from build123d import *

# Parameters (mm, degrees)
SKETCH1_W           = 260.096
SKETCH1_H           = 179.705
SKETCH1_W_2         = 1.524
SKETCH1_H_2         = 1.016
SKETCH1_W_3         = 1.3716
SKETCH1_W_4         = 1.397
SKETCH1_R           = 1.143
BOSS_EXTRUDE1_DEPTH = 3.048
BOSS_EXTRUDE2_DEPTH = 32.5374
SKETCH1_6_R         = 2.7686
SKETCH1_6_R_2       = 1.8415
BOSS_EXTRUDE3_DEPTH = 7.0104
BOSS_EXTRUDE4_DEPTH = 4.064
SKETCH1_8_R         = 3.9624
SKETCH1_8_R_2       = 1.651
BOSS_EXTRUDE5_DEPTH = 21.844
SKETCH3_W           = 254
SKETCH3_H           = 1.778
CUT_EXTRUDE1_DEPTH  = 0.508


# Read off the part's stored shape, not the designer's step: Boss-Extrude2
with BuildPart() as part:
    # Sketch1 → Boss-Extrude1 (new body)
    with BuildSketch(Plane.XY):
        Rectangle(SKETCH1_W, SKETCH1_H)
        with Locations((-126.238, -85.6615)):
            Rectangle(SKETCH1_W_2, SKETCH1_H_2, mode=Mode.SUBTRACT)
        with Locations((-126.3142, -58.2676)):
            Rectangle(SKETCH1_W_3, SKETCH1_H_2, mode=Mode.SUBTRACT)
        with Locations((-126.3142, -55.2704)):
            Rectangle(SKETCH1_W_3, SKETCH1_H_2, mode=Mode.SUBTRACT)
        with Locations((-126.3015, -20.4216)):
            Rectangle(SKETCH1_W_4, SKETCH1_H_2, mode=Mode.SUBTRACT)
        with Locations((-126.3015, -17.4244)):
            Rectangle(SKETCH1_W_4, SKETCH1_H_2, mode=Mode.SUBTRACT)
        with Locations(Location((-113.9952, -68.9864, 0), (0, 0, 180))):
            Circle(SKETCH1_R, mode=Mode.SUBTRACT)
        with Locations((-126.3015, 17.4244)):
            Rectangle(SKETCH1_W_4, SKETCH1_H_2, mode=Mode.SUBTRACT)
        with Locations((-126.3015, 20.4216)):
            Rectangle(SKETCH1_W_4, SKETCH1_H_2, mode=Mode.SUBTRACT)
        with Locations((-126.3015, 55.2704)):
            Rectangle(SKETCH1_W_4, SKETCH1_H_2, mode=Mode.SUBTRACT)
        with Locations((-126.3015, 58.2676)):
            Rectangle(SKETCH1_W_4, SKETCH1_H_2, mode=Mode.SUBTRACT)
    extrude(amount=BOSS_EXTRUDE1_DEPTH)

    # Boss-Extrude2 outline → Boss-Extrude2 (add)
    with BuildSketch(Plane.XY):
        Polygon((-127, -87.9475), (-127, -86.1695), (-125.476, -86.1695), (-125.476, -85.1535), (-127, -85.1535), (-127, 85.1535), (-125.476, 85.1535), (-125.476, 86.1695), (-127, 86.1695), (-127, 87.9475), (-125.476, 87.9475), (-127, 89.8525), (-130.048, 89.8525), (-130.048, -89.8525), (-127, -89.8525), (-125.476, -87.9475), align=None)
        Polygon((125.476, -87.9475), (127, -89.8525), (130.048, -89.8525), (130.048, 89.8525), (127, 89.8525), (125.476, 87.9475), (127, 87.9475), (127, 86.1695), (125.476, 86.1695), (125.476, 85.1535), (127, 85.1535), (127, -85.1535), (125.476, -85.1535), (125.476, -86.1695), (127, -86.1695), (127, -87.9475), align=None)
    extrude(amount=BOSS_EXTRUDE2_DEPTH)

    # Sketch1_6 → Boss-Extrude3 (add)
    # profile 1 of 8: a face of its own
    with BuildSketch(Plane.XY):
        with Locations((-113.9952, -68.9864)):
            Circle(SKETCH1_6_R)
        with Locations((-113.9952, -68.9864)):
            Circle(SKETCH1_6_R_2, mode=Mode.SUBTRACT)
    # profile 2 of 8: a face of its own
    with BuildSketch(Plane.XY):
        with Locations((-37.8968, -68.9864)):
            Circle(SKETCH1_6_R)
        with Locations((-37.8968, -68.9864)):
            Circle(SKETCH1_6_R_2, mode=Mode.SUBTRACT)
    # profile 3 of 8: a face of its own
    with BuildSketch(Plane.XY):
        with Locations((38.2016, 68.9864)):
            Circle(SKETCH1_6_R)
        with Locations((38.2016, 68.9864)):
            Circle(SKETCH1_6_R_2, mode=Mode.SUBTRACT)
    # profile 4 of 8: a face of its own
    with BuildSketch(Plane.XY):
        Circle(SKETCH1_6_R)
        Circle(SKETCH1_6_R_2, mode=Mode.SUBTRACT)
    # profile 5 of 8: a face of its own
    with BuildSketch(Plane.XY):
        with Locations((38.2016, -68.9864)):
            Circle(SKETCH1_6_R)
        with Locations((38.2016, -68.9864)):
            Circle(SKETCH1_6_R_2, mode=Mode.SUBTRACT)
    # profile 6 of 8: a face of its own
    with BuildSketch(Plane.XY):
        with Locations((-113.9952, 68.9864)):
            Circle(SKETCH1_6_R)
        with Locations((-113.9952, 68.9864)):
            Circle(SKETCH1_6_R_2, mode=Mode.SUBTRACT)
    # profile 7 of 8: a face of its own
    with BuildSketch(Plane.XY):
        with Locations((-119.9896, 0)):
            Circle(SKETCH1_6_R)
        with Locations((-119.9896, 0)):
            Circle(SKETCH1_6_R_2, mode=Mode.SUBTRACT)
    # profile 8 of 8: a face of its own
    with BuildSketch(Plane.XY):
        with Locations((-37.8968, 68.9864)):
            Circle(SKETCH1_6_R)
    extrude(amount=BOSS_EXTRUDE3_DEPTH)

    # Sketch1_7 → Boss-Extrude4 (add)
    with BuildSketch(Plane.XY):
        Polygon((125.476, -86.1695), (125.476, -85.1535), (79.460364238, -85.1535), (-125.476, -85.1535), (-125.476, -86.1695), (78.870243492, -86.1695), align=None)
        Polygon((-125.476, -87.9475), (-127, -89.8525), (127, -89.8525), (125.476, -87.9475), (77.837532187, -87.9475), align=None)
        Polygon((-127, 89.8525), (-125.476, 87.9475), (77.048819747, 87.9475), (125.476, 87.9475), (127, 89.8525), align=None)
        Polygon((-125.476, 86.1695), (-125.476, 85.1535), (79.071493661, 85.1535), (125.476, 85.1535), (125.476, 86.1695), (78.335975874, 86.1695), align=None)
    extrude(amount=BOSS_EXTRUDE4_DEPTH)

    # Sketch1_8 → Boss-Extrude5 (add)
    # profile 1 of 2: a face of its own
    with BuildSketch(Plane.XY):
        with Locations((-119.9134, -78.6765)):
            Circle(SKETCH1_8_R)
        with Locations((-119.9134, -78.6765)):
            Circle(SKETCH1_8_R_2, mode=Mode.SUBTRACT)
    # profile 2 of 2: a face of its own
    with BuildSketch(Plane.XY):
        with Locations((-119.9134, 78.6765)):
            Circle(SKETCH1_8_R)
        with Locations((-119.9134, 78.6765)):
            Circle(SKETCH1_8_R_2, mode=Mode.SUBTRACT)
    extrude(amount=BOSS_EXTRUDE5_DEPTH)

    # Sketch3 → Cut-Extrude1 (cut)
    with BuildSketch(Plane.XY.offset(3.048)):
        with Locations((0, 87.0585)):
            Rectangle(SKETCH3_W, SKETCH3_H)
        with Locations((0, -87.0585)):
            Rectangle(SKETCH3_W, SKETCH3_H)
    extrude(amount=-CUT_EXTRUDE1_DEPTH, mode=Mode.SUBTRACT)


solid = part.part
CAD build for the part. Positions are in the model's coordinates, mm. A direction names the side the tool comes from. Coordinates: 2 decimals unless noted, no trailing zeros. Write each loop counter-clockwise with the first axis right and the second up, starting at its lowest first coordinate (ties: lowest second). Pieces come first, ordered by that corner, then holes. Notation, with made-up numbers: M -4,-13.75 L 5,-13.75 A37 cw 5,25.25 Z; hole C 40,-19 d9. An arc over 180 degrees is marked long. Answer as a JSON object with one key per item and string values. Group by question number.
1) Pin check, flat tips, straight feed: pin 1 Ø10 at (x, y) = (-61.5, -25) entering from +Z; pin 2 Ø5 at (x, z) = (51.5, 8) entering from +Y; pin 3 Ø3 at (x, y) = (-0.5, 0.5) entering from +Z; pin 4 Ø1.4 at (x, y) = (-46, -87) entering from +Z. Stop position of each tip, or through.
2) Saw through at B-B (y = -36). Write the cut outline in (x, z), plus the area to 3 significant figures.
3) Saw through at C-C (x = -7). Write the cut outline in (y, z), plus the area to 3 significant figures.
4) Tool access for faces 1 (the face through (-118, -79, 21.844)), 2 (the face through (1, 86.17, 3)), 3 (the face through (-130.048, -1, 16)): list every direction of +Z, -Z, +X, -X, +Y, -Y with a clear straight run to the whole face (end or side of a thin tool).
5) Mould opens along Y. For faces 4 (the face through (127, 1, 18)), 5 (the face through (-37, -71, 7.01)), 6 (the face through (-1, -89.852, 2)) say: +Y half, -Y half, draft (parallel to the pull), parting line (faces both ways), or undercut.
6) Wall check: line 1 (X direction, y = 0, z = 4); line 2 (X direction, y = -35, z = 30); line 3 (Z direction, x = 70, y = -43.5). Give the ranges that are in metal, low to high. Write a range as from..to.
Values follow:
{
 "1": {"pin 1": "stops at z = 3.05", "pin 2": "passes through", "pin 3": "stops at z = 7.01", "pin 4": "stops at z = 2.54"},
 "2": {"outline": "M -130.05,0 L 130.05,0 L 130.05,32.54 L 127,32.54 L 127,3.05 L -127,3.05 L -127,32.54 L -130.05,32.54 Z", "area": "973 mm2"},
 "3": {"outline": "M -89.85,0 L 89.85,0 L 89.85,4.06 L 87.95,4.06 L 87.95,2.54 L 86.17,2.54 L 86.17,4.06 L 85.15,4.06 L 85.15,3.05 L -85.15,3.05 L -85.15,4.06 L -86.17,4.06 L -86.17,2.54 L -87.95,2.54 L -87.95,4.06 L -89.85,4.06 Z", "area": "552 mm2"},
 "4": {"face 1": "+Z, +Y, -Y", "face 2": "+Z", "face 3": "+Z, -Z, -X, +Y, -Y"},
 "5": {"face 4": "undercut", "face 5": "draft", "face 6": "-Y half"},
 "6": {"line 1": "x = -130.05..-127, -122.76..-121.83, -118.15..-117.22, -2.77..-1.84, 1.84..2.77, 127..130.05", "line 2": "x = -130.05..-127, 127..130.05", "line 3": "z = 0..3.05"}
}
